For this review, take the finished solid that the model builds, in its own axes (mm). Face numbers are marked on the shaded views. A direction names the side the tool comes from. Coordinates: 2 decimals unless noted, no trailing zeros. Write each loop counter-clockwise with the first axis right and the second up, starting at its lowest first coordinate (ties: lowest second). Pieces come first, ordered by that corner, then holes. Notation, with made-up numbers: (-9.75, 15.5) -> (37.25, 15.5) arc R25 cw to (37.25, 43.5) -> close; hole circle Ø1 at (86, -35). An arc over 180 degrees is marked (long way). One line per item, written item: value. Start each with the question number.
1) For probe 1 along Z at (x, y) = (-30.5, -11); probe 2 along X at (y, z) = (-12, -4.5); probe 3 along X at (y, z) = (-1.5, -13.15), list the stretches that pass through material, from the lowest coordinate up. Write a range as from..to.
2) Add section A-A (z = -9.5). State the section outline as (x, y) points.
3) Mouldability with a two-part tool opening along X and no side actions: class the marked faces 1, 2 and 3 as released by +X, released by -X, zero draft, split by the parting line, or undercut.
4) For pin 1 Ø12 at (x, z) = (10, 8.5) entering from -Y; pin 2 Ø1.4 at (x, z) = (10.5, -12) entering from +Y; pin 3 Ø8 at (y, z) = (-12, -6.5) entering from -X; pin 4 Ø1 at (x, z) = (3, -11.5) entering from -Y, all flat-tipped, find the tip position at first contact; note any pin that passes through.
5) Add section B-B (x = 28). State the section outline as (y, z) points.
6) Machinability: for the marked faces 4, 5, 6 and 7, which of the approach directions +Z, -Z, +X, -X, +Y, -Y give a long, thin tool a straight path to every point of the face, cutting with its end or side? Answer none if there is none.
from build123d import *

# Parameters (mm, degrees)
F1_DEPTH = 20
F2_DEPTH = 1.2
F4_DEPTH = 30
F5_DEPTH = 1.2


with BuildPart() as f1:
    # F0 (on Front) → F1 (new body)
    with BuildSketch(Plane.XZ):
        with BuildLine():
            ThreePointArc((38.7, 12.5), (38.3485281374, 13.3485281374), (37.5, 13.7))
            Line((37.5, 13.7), (-37.5, 13.7))
            ThreePointArc((-37.5, 13.7), (-38.3485281374, 13.3485281374), (-38.7, 12.5))
            Line((-38.7, 12.5), (-38.7, -12.5))
            ThreePointArc((-38.7, -12.5), (-38.3485281374, -13.3485281374), (-37.5, -13.7))
            Line((-37.5, -13.7), (37.5, -13.7))
            ThreePointArc((37.5, -13.7), (38.3485281374, -13.3485281374), (38.7, -12.5))
            Line((38.7, -12.5), (38.7, 12.5))
        make_face()
        with BuildLine():
            Line((-36.3, 12.5), (36.3, 12.5))
            ThreePointArc((36.3, 12.5), (37.1485281374, 12.1485281374), (37.5, 11.3))
            Line((37.5, 11.3), (37.5, -11.3))
            ThreePointArc((37.5, -11.3), (37.1485281374, -12.1485281374), (36.3, -12.5))
            Line((36.3, -12.5), (-36.3, -12.5))
            ThreePointArc((-36.3, -12.5), (-37.1485281374, -12.1485281374), (-37.5, -11.3))
            Line((-37.5, -11.3), (-37.5, 11.3))
            ThreePointArc((-37.5, 11.3), (-37.1485281374, 12.1485281374), (-36.3, 12.5))
        make_face(mode=Mode.SUBTRACT)
    extrude(amount=F1_DEPTH)

    # F0 (on Front) → F2 (join)
    with BuildSketch(Plane.XZ):
        with BuildLine():
            ThreePointArc((37.5, 11.3), (37.1485281374, 12.1485281374), (36.3, 12.5))
            Line((36.3, 12.5), (-36.3, 12.5))
            ThreePointArc((-36.3, 12.5), (-37.1485281374, 12.1485281374), (-37.5, 11.3))
            Line((-37.5, 11.3), (-37.5, -11.3))
            ThreePointArc((-37.5, -11.3), (-37.1485281374, -12.1485281374), (-36.3, -12.5))
            Line((-36.3, -12.5), (36.3, -12.5))
            ThreePointArc((36.3, -12.5), (37.1485281374, -12.1485281374), (37.5, -11.3))
            Line((37.5, -11.3), (37.5, 11.3))
        make_face()
        with BuildLine():
            Line((-35.1000003621, 11.3000003621), (35.1000003621, 11.3000003621))
            ThreePointArc((35.1000003621, 11.3000003621), (35.9485284995, 10.9485284995), (36.3000003621, 10.1000003621))
            Line((36.3000003621, 10.1000003621), (36.3000003621, -10.1000003621))
            ThreePointArc((36.3000003621, -10.1000003621), (35.9485284995, -10.9485284995), (35.1000003621, -11.3000003621))
            Line((35.1000003621, -11.3000003621), (-35.1000003621, -11.3000003621))
            ThreePointArc((-35.1000003621, -11.3000003621), (-35.9485284995, -10.9485284995), (-36.3000003621, -10.1000003621))
            Line((-36.3000003621, -10.1000003621), (-36.3000003621, 10.1000003621))
            ThreePointArc((-36.3000003621, 10.1000003621), (-35.9485284995, 10.9485284995), (-35.1000003621, 11.3000003621))
        make_face(mode=Mode.SUBTRACT)
    extrude(amount=F2_DEPTH)

    # F3 (on face) → F4 (cut)
    with BuildSketch(Plane(origin=(0, 0, -13.7), x_dir=(1, 0, 0), z_dir=(0, 0, -1))):
        with BuildLine():
            Line((-37.5, 0), (-37.5, 3.9494897428))
            ThreePointArc((-37.5, 3.9494897428), (-40.3371173071, 0.6123724357), (-36, 0))
            Line((-36, 0), (-37.5, 0))
        make_face()
        with BuildLine():
            ThreePointArc((-36, 0), (-35.6282917549, 0.709430585), (-35.5, 1.5))
            ThreePointArc((-35.5, 1.5), (-36.0635083269, 3.0811388301), (-37.5, 3.9494897428))
            Line((-37.5, 3.9494897428), (-37.5, 0))
            Line((-37.5, 0), (-36, 0))
        make_face()
        with BuildLine():
            ThreePointArc((37.5, 3.9494897428), (35.6628826929, 2.3876275643), (36, 0))
            Line((36, 0), (37.5, 0))
            Line((37.5, 0), (37.5, 3.9494897428))
        make_face()
        with BuildLine():
            Line((37.5, 0), (36, 0))
            ThreePointArc((36, 0), (38.790569415, -0.8717082451), (40.5, 1.5))
            ThreePointArc((40.5, 1.5), (39.5811388301, 3.4364916731), (37.5, 3.9494897428))
            Line((37.5, 3.9494897428), (37.5, 0))
        make_face()
    extrude(amount=-F4_DEPTH, mode=Mode.SUBTRACT)

    # F3 (on face) → F5 (join)
    with BuildSketch(Plane(origin=(0, 0, -13.7), x_dir=(1, 0, 0), z_dir=(0, 0, -1))):
        with BuildLine():
            ThreePointArc((-36, 0), (-40.3371173071, 0.6123724357), (-37.5, 3.9494897428))
            Line((-37.5, 3.9494897428), (-37.5, 6.9772255751))
            ThreePointArc((-37.5, 6.9772255751), (-42.5338498913, -1.6135518565), (-32.7084973779, 0))
            Line((-32.7084973779, 0), (-36, 0))
        make_face()
    extrude(amount=-F5_DEPTH)


solid = f1.part
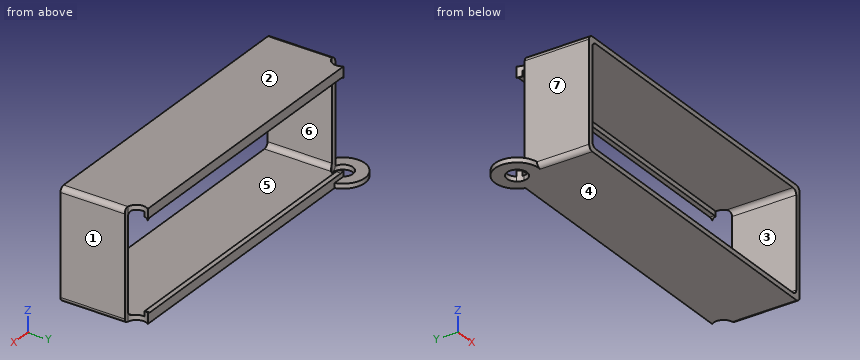
Numbers:
1. probe 1: -13.7..-12.5, 12.5..13.7
1. probe 2: -38.7..-37.5, 37.5..38.7
1. probe 3: -43.5..-40.5, -35.5..35.5
2. outline: (-38.7, -20) -> (-37.5, -20) -> (-37.5, -3.95) arc R2.5 cw to (-38.7, -3.9) -> close; (37.5, -20) -> (38.7, -20) -> (38.7, -3.9) arc R2.5 cw to (37.5, -3.95) -> close
3. face 1: released by +X
3. face 2: zero draft
3. face 3: undercut
4. pin 1: y = -20
4. pin 2: y = 0
4. pin 3: x = -38.7
4. pin 4: y = -1.2
5. outline: (-20, -13.7) -> (0, -13.7) -> (0, -11.3) -> (-1.2, -11.3) -> (-1.2, -12.5) -> (-20, -12.5) -> close; (-20, 12.5) -> (-1.2, 12.5) -> (-1.2, 11.3) -> (0, 11.3) -> (0, 13.7) -> (-20, 13.7) -> close
6. face 4: -Z, +X, -X, +Y, -Y
6. face 5: -Y
6. face 6: +Y, -Y
6. face 7: +Z, -X, +Y, -Y
